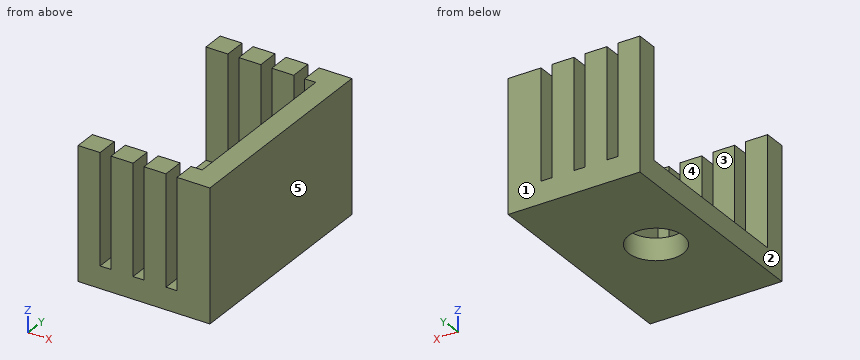
```python
from build123d import *

# Parameters (mm, degrees)
F0_W     = 12
F0_H     = 20
F1_DEPTH = 2
F2_W     = 2
F2_H     = 2
F2_H_2   = 8
F3_DEPTH = 10
F4_R     = 2.5
F5_DEPTH = 25
F6_DEPTH = 10


with BuildPart() as f1:
    # F0 (on Top) → F1 (new body)
    with BuildSketch(Plane.XY):
        with Locations((-6, 10)):
            Rectangle(F0_W, F0_H)
    extrude(amount=F1_DEPTH)

    # F2 (on face) → F3 (join)
    with BuildSketch(Plane.XY.offset(2)):
        with Locations((-11, 19)):
            Rectangle(F2_W, F2_H)
        Polygon((0, 20), (-3, 20), (-3, 18), (-2, 18), (0, 18), align=None)
        with Locations((-5, 19)):
            Rectangle(F2_W, F2_H)
        with Locations((-8, 19)):
            Rectangle(F2_W, F2_H)
        with Locations((-1, 14)):
            Rectangle(F2_W, F2_H_2)
        with Locations((-1, 6)):
            Rectangle(F2_W, F2_H_2)
        with Locations((-11, 1)):
            Rectangle(F2_W, F2_H)
        with Locations((-8, 1)):
            Rectangle(F2_W, F2_H)
    extrude(amount=F3_DEPTH)

    # F4 (on face) → F5 (cut)
    with BuildSketch(Plane.XY.offset(2)):
        with Locations((-7, 10)):
            Circle(F4_R)
    extrude(amount=-F5_DEPTH, mode=Mode.SUBTRACT)

    # F2 (on face) → F6 (join)
    with BuildSketch(Plane.XY.offset(2)):
        with Locations((-5, 1)):
            Rectangle(F2_W, F2_H)
        Polygon((0, 2), (-2, 2), (-3, 2), (-3, 0), (0, 0), align=None)
    extrude(amount=F6_DEPTH)


solid = f1.part
```
Design review of the part built by this model. Coordinates are the model's own, in mm. Face numbers are marked on the shaded views. A direction names the side the tool comes from. Give positions to 0.01 mm unless a question says otherwise; leave off trailing zeros. Write each loop counter-clockwise with the first axis right and the second up, starting at its lowest first coordinate (ties: lowest second). Pieces come first, ordered by that corner, then holes. Notation, with made-up numbers: (-22.5, 10.25) - (22.5, 10.25) arc R15 cw to (22.5, 16.25) - close; hole circle Ø10 at (-37.75, -34). An arc over 180 degrees is marked (long way). Return JSON: item names as keys, results as strings. Group by question number.
(1) Mouldability with a two-part tool opening along Y and no side actions: class the marked faces 1, 2 and 3 as +Y half, -Y half, draft (parallel to the pull), parting line (faces both ways), or undercut.
(2) We need section D-D, the plane y = 13.5. Give the boundary of the cut face in (x, z).
(3) To check wall thickness, follow probe 1 along X at (y, z) = (18.5, 5); probe 2 along Y at (x, z) = (-7, 0.4); probe 3 along Y at (x, z) = (-5.5, 9). State the ranges of each line that lie inside material, in increasing order.
(4) Machinability: for the marked faces 4 and 5, which of the approach directions +Z, -Z, +X, -X, +Y, -Y give a long, thin tool a straight path to every point of the face, cutting with its end or side? Answer none if there is none.
(5) We need section C-C, the plane z = 3. Give the number of separate pieces and of enclosed holes in the cut face, then the cut area to 3 significant figures.
(6) We need section A-A, the plane x = -8.5. Give the boundary of the cut face in (y, z).
(7) Insertion check: pin 1 (3 mm diameter, centred on y = 8.5, z = 7.5, fed in from -X). The pin has a flat end and moves straight along its axis. Give the tip position at first contact, or say it passes through.
(8) We need section B-B, the plane y = 10. Give the boundary of the cut face in (x, z), then the cut area to 3 significant figures.
Reported:
{
 "1": {"face 1": "+Y half", "face 2": "draft", "face 3": "undercut"},
 "2": {"outline": "(-12, 0) - (0, 0) - (0, 12) - (-2, 12) - (-2, 2) - (-12, 2) - close"},
 "3": {"probe 1": "x = -12 to -10, -9 to -7, -6 to -4, -3 to 0", "probe 2": "y = 0 to 7.5, 12.5 to 20", "probe 3": "y = 0 to 2, 18 to 20"},
 "4": {"face 4": "+Z, -X", "face 5": "+Z, -Z, +X, +Y, -Y"},
 "5": {"separate pieces": "7", "enclosed holes": "0", "area": "68.0 mm2"},
 "6": {"outline": "(0, 0) - (8, 0) - (8, 2) - (2, 2) - (2, 12) - (0, 12) - close; (12, 0) - (20, 0) - (20, 12) - (18, 12) - (18, 2) - (12, 2) - close"},
 "7": {"pin 1": "stops at x = -2"},
 "8": {"outline": "(-12, 0) - (-9.5, 0) - (-9.5, 2) - (-12, 2) - close; (-4.5, 0) - (0, 0) - (0, 12) - (-2, 12) - (-2, 2) - (-4.5, 2) - close", "area": "34.0 mm2"}
}
